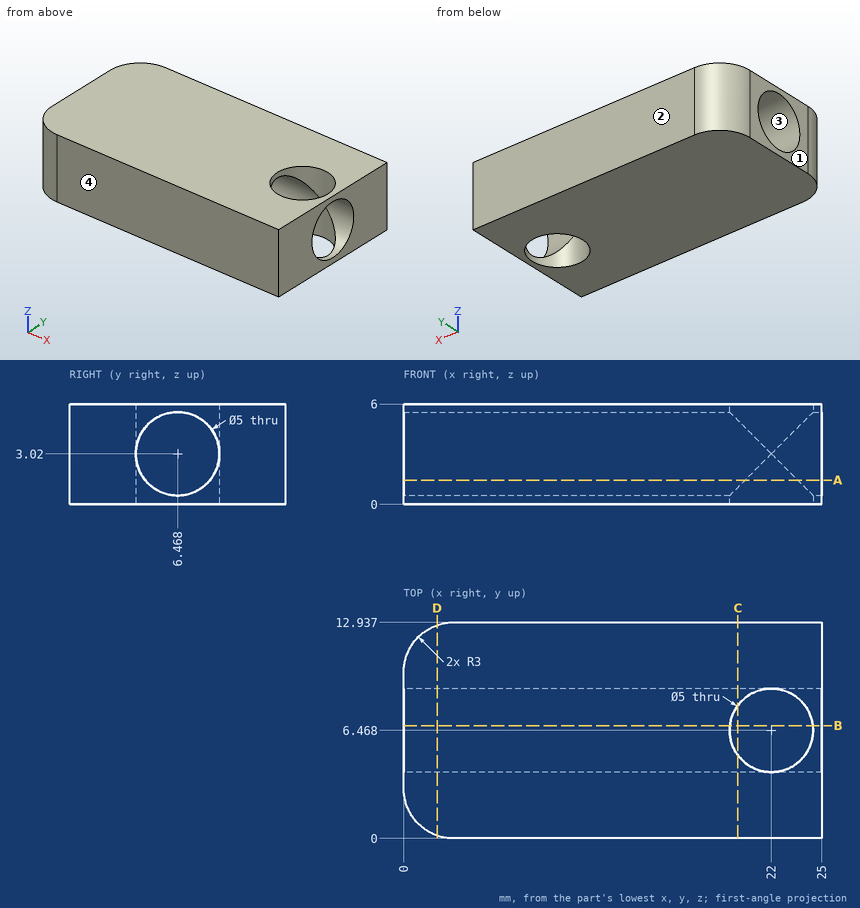
The figure shows three views and two pictorial views of one solid part (mm, origin at its lowest corner). Answer the questions. Give positions to 0.01 mm unless a question says otherwise; leave off trailing zeros. Loops run counter-clockwise (first coordinate to the right, second up) from the corner with the lowest first, then second, coordinate; pieces in that order, holes last. Notation, with made-up numbers: (85.5, -33.75) - (116.5, -33.75) arc R15 cw to (116.5, -9.75) - close; hole circle Ø2 at (-23, -3). An arc over 180 degrees is marked (long way). Answer in a Markdown table with one row per item.
(1) Consider L1, parallel to Y at x = 16.5, z = 2.95; L2, parallel to Z at x = 10.25, y = 6.5; L3, parallel to Y at x = 12, z = 3.8 (1 decimal). Determine where each line is inside the solid, lowest interval first. Write a range as [from, to].
Results list:
| item | result |
|---|---|
| L1 | y = [0, 3.97], [8.97, 12.94] |
| L2 | z = [0, 0.52], [5.52, 6] |
| L3 | y = [0, 4.1], [8.8, 12.9] |
(2) Section B-B (y = 6.75) is taken. Give the vertices of the cut face in (x, z) (1 decimal).
Results list:
| item | result |
|---|---|
| outline | (0, 0) - (19.5, 0) - (19.5, 0.5) - (0, 0.5) - close; (0, 5.5) - (19.5, 5.5) - (19.5, 6) - (0, 6) - close; (24.5, 0) - (25, 0) - (25, 0.5) - (24.5, 0.5) - close; (24.5, 5.5) - (25, 5.5) - (25, 6) - (24.5, 6) - close |
(3) A flat-ended cylindrical pin translates along its axis: pin 1 Ø4 at (x, y) = (22, 6.47) entering from +Z. Find the tip coordinate at first contact, or state that the pin passes through.
Results list:
| item | result |
|---|---|
| pin 1 | passes through |
(4) Section A-A (z = 1.45) is taken. Give the vertices of the cut face in (x, y) (1 decimal), and give its area (3 significant figures).
Results list:
| item | result |
|---|---|
| outline | (0, 3) arc R3 ccw to (3, 0) - (25, 0) - (25, 4.5) - (23.6, 4.5) arc R2.5 cw to (20.4, 4.5) - (0, 4.5) - close; (0, 8.4) - (20.4, 8.4) arc R2.5 cw to (23.6, 8.4) - (25, 8.4) - (25, 12.9) - (3, 12.9) arc R3 ccw to (0, 9.9) - close |
| area | 220 mm² |
(5) Section C-C (x = 20) is taken. Give the vertices of the cut face in (y, z).
Results list:
| item | result |
|---|---|
| outline | (0, 0) - (4.97, 0) - (4.97, 1.02) arc R2.5 cw to (4.97, 5.02) - (4.97, 6) - (0, 6) - close; (7.97, 0) - (12.94, 0) - (12.94, 6) - (7.97, 6) - (7.97, 5.02) arc R2.5 cw to (7.97, 1.02) - close |
(6) Section D-D (x = 2) is taken. Give the vertices of the cut face in (y, z) (1 decimal).
Results list:
| item | result |
|---|---|
| outline | (0.2, 0) - (12.8, 0) - (12.8, 6) - (0.2, 6) - close; hole circle Ø5 at (6.5, 3) |
(7) For a pull along Y with two mould halves and no side action, classify the marked faces 1, 2, 3 and 4 as pulls with the +Y half, pulls with the -Y half, needs draft (parallel to the pull), parting line crosses it, or undercut.
Results list:
| item | result |
|---|---|
| face 1 | needs draft |
| face 2 | pulls with the +Y half |
| face 3 | undercut |
| face 4 | pulls with the -Y half |
